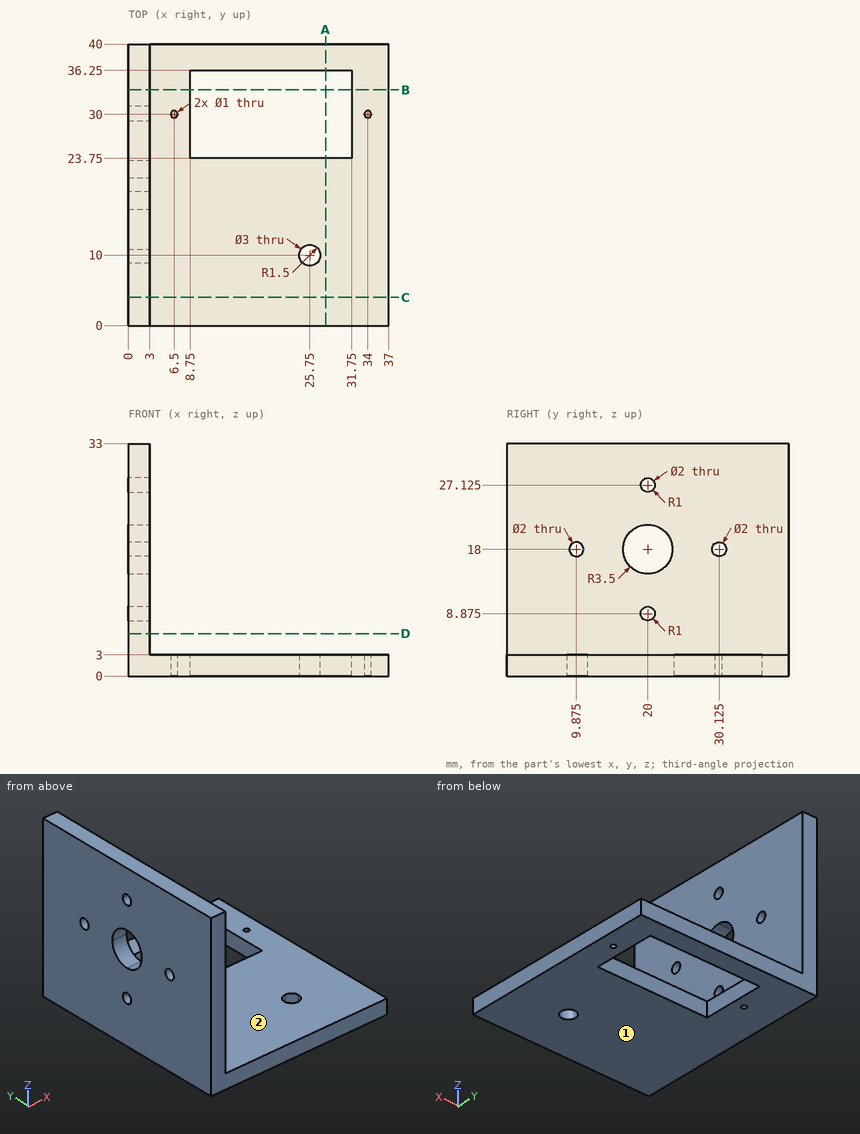
Geometry check sheet. Reference: drawing and pictorial views, mm from the part's lowest x, y, z. A direction names the side the tool comes from. Give positions to 0.01 mm unless a question says otherwise; leave off trailing zeros. Order: outer loops, then holes, each group sorted by start corner. A loop starts at its lowest first (then second) coordinate and runs counter-clockwise, first axis right, second up. Notation, with made-up numbers: M 25,46.5 L 37,46.5 A22 cw 37,69.5 Z; hole C -27,11 d6. An arc over 180 degrees is marked long. Answer as CSV lines item,"result". Start each with the question number.
Item 1: Tool access check on the marked faces 1 and 2. Record the directions out of +Z, -Z, +X, -X, +Y, -Y that give a thin tool (end or side, any length) a straight path to the whole face; none if there is none.
Item 2: Cross-section at C-C on y = 4. Enter the section's corners in (x, z).
Item 3: Cross-section at B-B on y = 33.5. Enter the section's corners in (x, z).
Item 4: Cross-section at D-D on z = 6. Enter the section's corners in (x, y), plus the area to 3 significant figures.
Item 5: Cross-section at A-A on x = 28. Enter the section's corners in (y, z), plus the area to 3 significant figures.
Item 6: Gauge pin test, flat ends, axial feed: P1, Ø1, axis at x = 27, y = 12, coming from the +Z side; P2, Ø3.5, axis at x = 22.5, z = 2, coming from the -Y side; P3, Ø12, axis at y = 14.5, z = 26, coming from the +X side. Record the tip position at first contact, or that the pin passes through.
Item 7: Thickness scan on line 1 (Y direction, x = 25.75, z = 2); line 2 (Y direction, x = 34, z = 0.7); line 3 (Z direction, x = 34, y = 19.5). Record the ranges inside material, lowest first. Write a range as [from, to].
Established:
1,face 1,"-Z, +X, -X, +Y, -Y"
1,face 2,"+Z, +X, +Y, -Y"
2,outline,"M 0,0 L 37,0 L 37,3 L 3,3 L 3,33 L 0,33 Z"
3,outline,"M 0,0 L 8.75,0 L 8.75,3 L 3,3 L 3,33 L 0,33 Z; M 31.75,0 L 37,0 L 37,3 L 31.75,3 Z"
4,outline,"M 0,0 L 3,0 L 3,40 L 0,40 Z"
4,area,"120 mm^2"
5,outline,"M 0,0 L 23.75,0 L 23.75,3 L 0,3 Z; M 36.25,0 L 40,0 L 40,3 L 36.25,3 Z"
5,area,"82.5 mm^2"
6,P1,"stops at z = 3"
6,P2,"stops at y = 0"
6,P3,"stops at x = 3"
7,line 1,"y = [0, 8.5], [11.5, 23.75], [36.25, 40]"
7,line 2,"y = [0, 29.5], [30.5, 40]"
7,line 3,"z = [0, 3]"
